For this review, use the dimensioned drawing (mm, ordinates from the lowest corner) and the shaded views. A direction names the side the tool comes from. Round coordinates to 2 decimals unless told otherwise and drop trailing zeros. Loops run counter-clockwise (first coordinate to the right, second up) from the corner with the lowest first, then second, coordinate; pieces in that order, holes last. Notation, with made-up numbers: (-25, 58) -> (30, 58) arc R22 ccw to (30, 83) -> close; hole circle Ø9 at (1.5, 32). An arc over 180 degrees is marked (long way). Answer as CSV lines item,"result". Start each with the question number.
(1) Take a section at A-A, the plane x = 21. Write out the cut boundary in (y, z), and give its area (3 significant figures).
(2) For P1, Ø1.8, axis at x = 9, y = 2.5, coming from the -Z side; P2, Ø4.5, axis at x = 52, z = 20, coming from the +Y side; P3, Ø2.5, axis at x = 50, y = 2.5, coming from the -Z side, all flat-tipped, find the tip position at first contact; note any pin that passes through.
(3) Take a section at C-C, the plane z = 32.5. Write out the cut boundary in (x, y).
(4) Machinability: for the marked faces 1, 2 and 3, which of the approach directions +Z, -Z, +X, -X, +Y, -Y give a long, thin tool a straight path to every point of the face, cutting with its end or side? Answer none if there is none.
(5) Take a section at D-D, the plane y = 7.25. State how many separate pieces and enclosed holes the cut face has, and give its area (3 significant figures).
(6) To check wall thickness, follow line 1 (X direction, y = 2, z = 51); line 2 (Z direction, x = 52, y = 3); line 3 (X direction, y = 6, z = 32.5). State the ranges of each line that lie inside material, in increasing order. Write a range as from..to.
(7) Take a section at B-B, the plane z = 19. Write out the cut boundary in (x, y), and give its area (3 significant figures).
(8) Draft analysis for pull direction Z (two halves, no side actions). For the marked faces 4, 5, 6 and 7, state which applies: +Z half, -Z half, draft (parallel to the pull), parting line (faces both ways), or undercut.
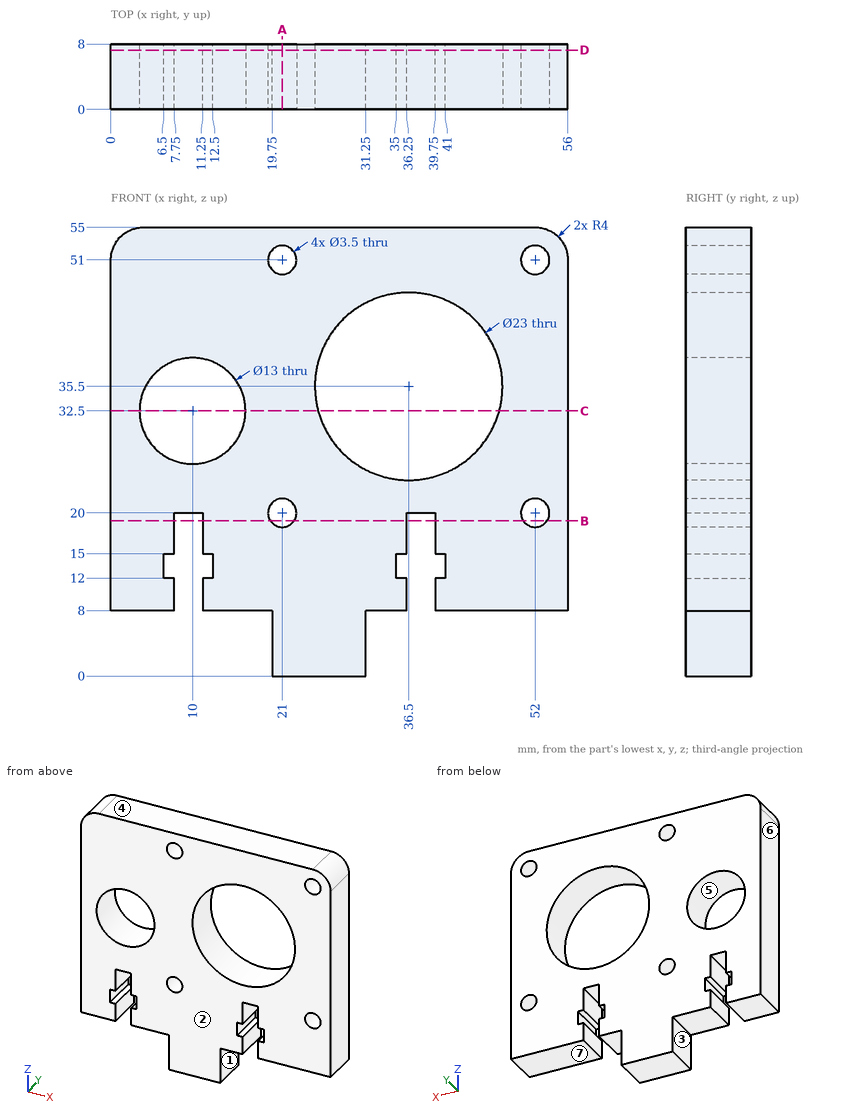
The answers:
1,outline,"(0, 0) -> (8, 0) -> (8, 18.25) -> (0, 18.25) -> close; (0, 21.75) -> (8, 21.75) -> (8, 49.25) -> (0, 49.25) -> close; (0, 52.75) -> (8, 52.75) -> (8, 55) -> (0, 55) -> close"
1,area,"384 mm²"
2,P1,"z = 20"
2,P2,"y = 8"
2,P3,"z = 8"
3,outline,"(0, 0) -> (3.5, 0) -> (3.5, 8) -> (0, 8) -> close; (16.5, 0) -> (25.4, 0) -> (25.4, 8) -> (16.5, 8) -> close; (47.6, 0) -> (56, 0) -> (56, 8) -> (47.6, 8) -> close"
4,face 1,"-Z, +X, +Y, -Y"
4,face 2,"+Z, -Z, +X, -X, -Y"
4,face 3,"-Z, -X, +Y, -Y"
5,separate pieces,"1"
5,enclosed holes,"6"
5,area,"2,030 mm²"
6,line 1,"0..19.25, 22.75..50.25, 53.75..56"
6,line 2,"8..18.25, 21.75..49.25, 52.75..55"
6,line 3,"0..3.5, 16.5..25.4, 47.6..56"
7,outline,"(0, 0) -> (7.75, 0) -> (7.75, 8) -> (0, 8) -> close; (11.25, 0) -> (19.56, 0) -> (19.56, 8) -> (11.25, 8) -> close; (22.44, 0) -> (36.25, 0) -> (36.25, 8) -> (22.44, 8) -> close; (39.75, 0) -> (50.56, 0) -> (50.56, 8) -> (39.75, 8) -> close; (53.44, 0) -> (56, 0) -> (56, 8) -> (53.44, 8) -> close"
7,area,"346 mm²"
8,face 4,"+Z half"
8,face 5,"undercut"
8,face 6,"draft"
8,face 7,"-Z half"
